Here's how the part is built. I have some questions about the finished solid (model axes, mm). Face numbers are marked on the shaded views. A direction names the side the tool comes from. Round coordinates to 2 decimals unless told otherwise and drop trailing zeros. Order: outer loops, then holes, each group sorted by start corner. A loop starts at its lowest first (then second) coordinate and runs counter-clockwise, first axis right, second up.
```python
from build123d import *

# Parameters (mm, degrees)
SKETCH1_R                = 2.5
SKETCH1_R_2              = 12.7
BOSS_EXTRUDE1_DEPTH      = 13.3
SKETCH1_3_R              = 2.5
BOSS_EXTRUDE2_DEPTH      = 16.3
BOSS_EXTRUDE2_DEPTH_BACK = 6.35
SKETCH2_R                = 3.175
BOSS_EXTRUDE3_DEPTH      = 20


with BuildPart() as part:
    # Sketch1 → Boss-Extrude1 (new body)
    with BuildSketch(Plane.XY):
        Circle(SKETCH1_R)
        Circle(SKETCH1_R_2)
        Circle(SKETCH1_R, mode=Mode.SUBTRACT)
    extrude(amount=BOSS_EXTRUDE1_DEPTH)

    # Sketch1_3 → Boss-Extrude2 (add, two sides)
    with BuildSketch(Plane.XY) as boss_extrude2_sk:
        Circle(SKETCH1_3_R)
    extrude(amount=BOSS_EXTRUDE2_DEPTH)
    extrude(boss_extrude2_sk.sketch, amount=-BOSS_EXTRUDE2_DEPTH_BACK)

    # Sketch2 → Boss-Extrude3 (add)
    with BuildSketch(Plane(origin=(0, 0, 0), x_dir=(0, 0, -1), z_dir=(1, 0, 0))):
        with Locations((-8.15, 0)):
            Circle(SKETCH2_R)
    extrude(amount=BOSS_EXTRUDE3_DEPTH)


solid = part.part
```
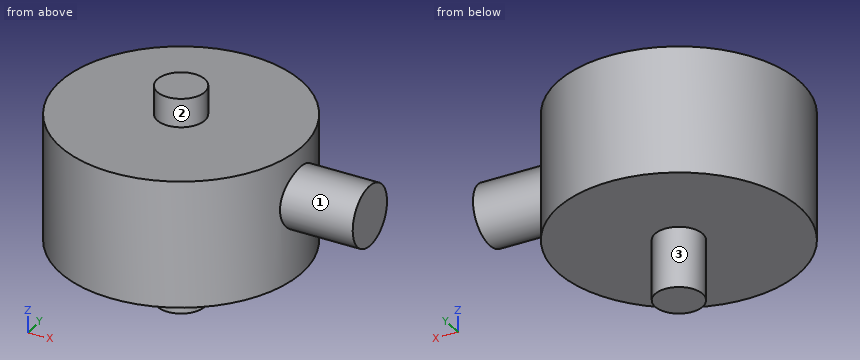
1. I'm going to push flat-ended pins straight in: P1, Ø1, axis at x = 9, z = 10.5, coming from the -Y side; P2, Ø3, axis at x = 5.5, y = 0.5, coming from the -Z side; P3, Ø1.5, axis at y = 2, z = -3.5, coming from the +X side. Where does each tip first touch, or does it pass through?
Evaluation:
P1: stops at y = -9.44
P2: stops at z = 0
P3: stops at x = 2.17
2. I need wall thicknesses on probe 1 along Z at (x, y) = (-2, 5.75); probe 2 along X at (y, z) = (2, 15.5); probe 3 along X at (y, z) = (9.25, 7.75). Which ranges of each line are inside material? Lowest first, please.
Evaluation:
probe 1: z = 0 to 13.3
probe 2: x = -1.5 to 1.5
probe 3: x = -8.7 to 8.7
3. If we section it at A-A, the plane x = 0: Write out the boundary of the cut face in (y, z), and give its area (3 significant figures).
Evaluation:
outline: (-12.7, 0) - (-2.5, 0) - (-2.5, -6.35) - (2.5, -6.35) - (2.5, 0) - (12.7, 0) - (12.7, 13.3) - (2.5, 13.3) - (2.5, 16.3) - (-2.5, 16.3) - (-2.5, 13.3) - (-12.7, 13.3) - close
area: 385 mm2
4. If we section it at B-B, the plane y = 0: Write out the boundary of the cut face in (x, z) (3 decimals), and give its area (3 significant figures).
Evaluation:
outline: (-12.7, 0) - (-2.5, 0) - (-2.5, -6.35) - (2.5, -6.35) - (2.5, 0) - (12.7, 0) - (12.7, 4.975) - (20, 4.975) - (20, 11.325) - (12.7, 11.325) - (12.7, 13.3) - (2.5, 13.3) - (2.5, 16.3) - (-2.5, 16.3) - (-2.5, 13.3) - (-12.7, 13.3) - close
area: 431 mm2
5. If we section it at D-D, the plane z = -2.75: Write out the boundary of the cut face in (x, y).
Evaluation:
outline: circle Ø5 at (0, 0)
6. On a 3-axis mill with a long thin cutter (end or side, diameter ignored), from which of +Z, -Z, +X, -X, +Y, -Y can I reach the whole of each face in a straight line? I mean the marked faces 1, 2 and 3. Say none if no direction works.
Evaluation:
face 1: +X
face 2: +Z
face 3: -Z
7. If we section it at C-C, the plane z = 8.15: Write out the boundary of the cut face in (x, y) (3 decimals), and give its area (3 significant figures).
Evaluation:
outline: (12.297, -3.175) - (20, -3.175) - (20, 3.175) - (12.297, 3.175) arc R12.7 ccw (long way) to start
area: 554 mm2
